Build history of the part. All positions in model axes, mm. A direction names the side the tool comes from. Give positions to 0.01 mm unless a question says otherwise; leave off trailing zeros. Write each loop counter-clockwise with the first axis right and the second up, starting at its lowest first coordinate (ties: lowest second). Pieces come first, ordered by that corner, then holes. Notation, with made-up numbers: M -35,81 L 7,81 A36 cw 7,120 Z; hole C 83.25,35 d3. An arc over 180 degrees is marked long. One line per item, written item: value. Start each with the question number.
Autodesk Inventor part; units mm, degrees
ref_plane "YZ Plane" through (0, 0, 0) normal (1, 0, 0) x (0, 1, 0)
ref_plane "XZ Plane" through (0, 0, 0) normal (0, 1, 0) x (-1, 0, 0)
ref_plane "XY Plane" through (0, 0, 0) normal (0, 0, 1) x (1, 0, 0)
sketch "Sketch1" plane through (0, 0, 0) normal (0, 0, 1) x (1, 0, 0)
  line L0 (0, -3.85) -> (0, 3.85)
  line L1 (-1.45, 0) -> (8.7, 0)
  line L2 (4.18, -2.75) -> (4.18, 2.75)
  line L3 (4.18, 2.75) -> (7.25, 2.75)
  line L4 (7.25, 2.75) -> (7.25, 2)
  line L5 (7.25, 2) -> (4.945, 2)
  line L6 (4.945, 2) -> (4.945, -2)
  line L7 (4.945, -2) -> (7.25, -2)
  line L8 (7.25, -2) -> (7.25, -2.75)
  line L9 (7.25, -2.75) -> (4.18, -2.75)
  point P0 (0, 0)
  point P1 (4.945, 0)
  dimension "d0" = 8.36
  dimension "d1" = 9.89
  dimension "d2" = 14.5
  dimension "d3" = 0.75
  dimension "d4" = 4
  dimension "d5" = 0.75
revolve "Revolution1" add sketch "Sketch1" angle 360 about axis through (0, -10, 0) along (0, 1, 0)
sketch "Sketch3" plane through (0, 2.75, 0) normal (0, 1, 0) x (1, 0, 0)
  circle A0 centre (0, 0) radius 7.25
  circle A1 centre (0, 0) radius 4.18
  line L0 (-10.15, 0) -> (10.15, 0)
  line L1 (0, 10.15) -> (0, -10.15)
  line L2 (4.1788, 0.1015) -> (7.1928, 0.9091)
  line L3 (4.1788, -0.1015) -> (7.1928, -0.9091)
  arc A2 (4.1788, -0.1015) -> (4.1788, 0.1015) centre (0, 0) ccw
  arc A3 (7.1928, -0.9091) -> (7.1928, 0.9091) centre (0, 0) ccw
  dimension "d15" = 15
  dimension "d16" = 30
  dimension "d17" = 3.014
  dimension "d18" = 3.014
extrude "Extrusion2" cut sketch "Sketch3" against normal through all contours L0 A1 L2 A0 | A0 L3 A1 L0
equation "\"d3\" = d5"
properties part number "311-04" material "Brass, Soft Yellow"
1) Band-saw the part on A-A (z = 3.75). List the corners of the cut face in (x, y).
2) Band-saw the part on C-C (z = 6). List the corners of the cut face in (x, y).
3) Tool access for faces 1 (the face through (4.66, 0.04, 0.23)), 2 (the face through (3.1, 2.75, 3.1)), 3 (the face through (-2, 2, 5)): list every direction of +Z, -Z, +X, -X, +Y, -Y with a clear straight run to the whole face (end or side of a thin tool).
4) Probe line 1 along Z through (x, y) = (0, -0.85) (3 decimals); line 2 along Y through (x, z) = (-4.5, -3.25); line 3 along X through (y, z) = (1.45, 1.75). List the from-to ranges inside material, lowest first. Write a range as from..to.
5) Mould opens along X. For faces 4 (the face through (-2, -2, 5)), 5 (the face through (-4.176, 0.038, -0.182)), 6 (the face through (-7.244, -2.38, 0.306)), 7 (the face through (4.66, 0.04, -0.23)) say: released by +X, released by -X, zero draft, split by the parting line, or undercut.
6) Band-saw the part on B-B (x = 0). List the corners of the cut face in (y, z) (3 decimals).
7) Drop flat-ended pins along their axis: P1, Ø4.5, axis at x = -3, z = 1.5, coming from the +Y side; P2, Ø1.5, axis at x = -1.5, y = -1.5, coming from the -Z side. Give the stop position or say it passes through.
Model answer:
1. outline: M -6.2,-2.75 L -1.85,-2.75 L -1.85,2.75 L -6.2,2.75 L -6.2,2 L -3.22,2 L -3.22,-2 L -6.2,-2 Z; M 1.85,-2.75 L 6.2,-2.75 L 6.2,-2 L 3.22,-2 L 3.22,2 L 6.2,2 L 6.2,2.75 L 1.85,2.75 Z
2. outline: M -4.07,-2.75 L 4.07,-2.75 L 4.07,-2 L -4.07,-2 Z; M -4.07,2 L 4.07,2 L 4.07,2.75 L -4.07,2.75 Z
3. face 1: +X, +Y, -Y
3. face 2: +Z, -Z, +X, -X, +Y
3. face 3: none
4. line 1: z = -4.945..-4.18, 4.18..4.945
4. line 2: y = -2.75..-2, 2..2.75
4. line 3: x = -4.62..-3.8, 3.8..4.62
5. face 4: zero draft
5. face 5: undercut
5. face 6: split by the parting line
5. face 7: released by +X
6. outline: M -2.75,-7.25 L -2,-7.25 L -2,-4.945 L 2,-4.945 L 2,-7.25 L 2.75,-7.25 L 2.75,-4.18 L -2.75,-4.18 Z; M -2.75,4.18 L 2.75,4.18 L 2.75,7.25 L 2,7.25 L 2,4.945 L -2,4.945 L -2,7.25 L -2.75,7.25 Z
7. P1: stops at y = 2.75
7. P2: stops at z = -7.19
